Geometry check sheet. Reference: drawing and pictorial views, mm from the part's lowest x, y, z. A direction names the side the tool comes from. Coordinates: 2 decimals unless noted, no trailing zeros. Loops run counter-clockwise (first coordinate to the right, second up) from the corner with the lowest first, then second, coordinate; pieces in that order, holes last.
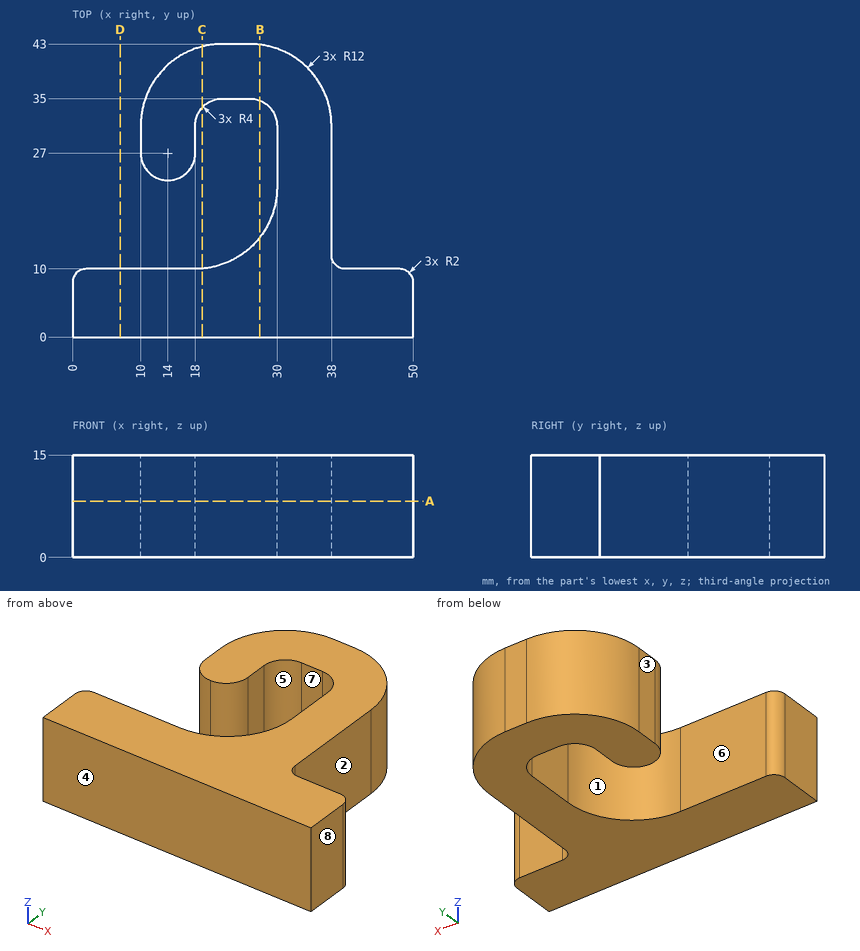
1) Section check A-A on z = 8.25. Record the cut outline in (x, y), and give its area (3 significant figures).
Data:
outline: (0, 0) - (50, 0) - (50, 8) arc R2 ccw to (48, 10) - (40, 10) arc R2 cw to (38, 12) - (38, 31) arc R12 ccw to (26, 43) - (22, 43) arc R12 ccw to (10, 31) - (10, 27) arc R4 ccw to (18, 27) - (18, 31) arc R4 cw to (22, 35) - (26, 35) arc R4 cw to (30, 31) - (30, 22) arc R12 cw to (18, 10) - (2, 10) arc R2 ccw to (0, 8) - close
area: 988 mm2
2) Access from +Z, -Z, +X, -X, +Y, -Y to the whole of each face (thin tool, end or side, straight path). Record for the marked faces 1, 2, 3, 4 and 5.
Data:
face 1: +Z, -Z, -X
face 2: +Z, -Z, +X, +Y
face 3: +Z, -Z, -X, +Y
face 4: +Z, -Z, +X, -X, -Y
face 5: +Z, -Z
3) Section check C-C on x = 19. Record the cut outline in (y, z), and give its area (3 significant figures).
Data:
outline: (0, 0) - (10.04, 0) - (10.04, 15) - (0, 15) - close; (33.65, 0) - (42.62, 0) - (42.62, 15) - (33.65, 15) - close
area: 285 mm2
4) Depth check by flat-ended pin: pin 1 (4 mm diameter, centred on x = 42.5, z = 11, fed in from +Y); pin 2 (5 mm diameter, centred on y = 21.5, z = 13, fed in from -X); pin 3 (3 mm diameter, centred on x = 17, z = 5.5, fed in from +Y). Enter the tip coordinate at first touch or a pass-through.
Data:
pin 1: stops at y = 10
pin 2: stops at x = 11.35
pin 3: stops at y = 42.48
5) Material ranges on probe 1 along X at (y, z) = (31, 10.5); probe 2 along Y at (x, z) = (21.5, 4.5); probe 3 along X at (y, z) = (26, 10.5), recorded low to high.
Data:
probe 1: x = 10 to 18, 30 to 38
probe 2: y = 0 to 10.52, 34.97 to 42.99
probe 3: x = 10.13 to 17.87, 30 to 38
6) Section check D-D on x = 7. Record the cut outline in (y, z), and give its area (3 significant figures).
Data:
outline: (0, 0) - (10, 0) - (10, 15) - (0, 15) - close
area: 150 mm2
7) Mould release check, pull along X, two halves, no side actions. Record for the marked faces 6, 7 and 8: +X half, -X half, draft (parallel to the pull), parting line (faces both ways), or undercut.
Data:
face 6: draft
face 7: undercut
face 8: +X half
8) Section check B-B on x = 27.5. Record the cut outline in (y, z).
Data:
outline: (0, 0) - (14.67, 0) - (14.67, 15) - (0, 15) - close; (34.71, 0) - (42.91, 0) - (42.91, 15) - (34.71, 15) - close
